from build123d import *

# Parameters (mm, degrees)
SKETCH_1_W      = 289
SKETCH_1_H      = 22.5
EXTRUDE_1_DEPTH = 21
FILLET_1_R      = 9


with BuildPart() as part:
    # 草图1 → 凸台-拉伸1 (new body)
    with BuildSketch(Plane.XY):
        Rectangle(SKETCH_1_W, SKETCH_1_H)
    extrude(amount=EXTRUDE_1_DEPTH)

    # 圆角1
    fillet_1_edges = [part.edges().sort_by_distance(p)[0] for p in [
        (0, 11.25, 0),
    ]]
    fillet(fillet_1_edges, radius=FILLET_1_R)


solid = part.part
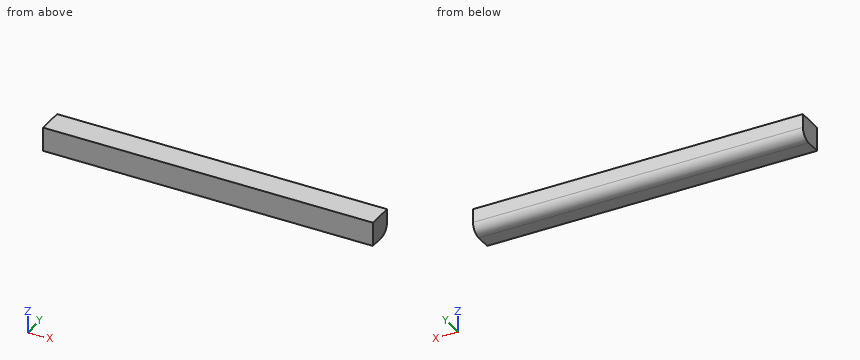
Could you check a few things on this model? Use its own coordinates, in mm. Round coordinates to 2 decimals unless told otherwise and drop trailing zeros. Order: outer loops, then holes, each group sorted by start corner. A loop starts at its lowest first (then second) coordinate and runs counter-clockwise, first axis right, second up. Notation, with made-up numbers: M 17,-32.5 L 59,-32.5 A13 ccw 59,-17.5 Z; hole C 56,-31.75 d10. An arc over 180 degrees is marked long. One line per item, written item: value.
(1) I'm going to push flat-ended pins straight in: P1, Ø4, axis at x = 38.5, z = 4, coming from the +Y side; P2, Ø10, axis at x = -87.5, y = 7, coming from the -Z side. Where does each tip first touch, or does it pass through?
Ans:
P1: stops at y = 10.74
P2: stops at z = 0
(2) Imagine slicing it at B-B (y = 8.75). Write out the boundary of the cut face in (x, z), and give its area (3 significant figures).
Ans:
outline: M -144.5,2.78 L 144.5,2.78 L 144.5,21 L -144.5,21 Z
area: 5,270 mm^2
(3) I need wall thicknesses on line 1 along Z through (x, y) = (-58, 3); line 2 along Z through (x, y) = (-33, 3.25); line 3 along Y through (x, z) = (40.5, 6.25). Which ranges of each line are inside material? Lowest first, please. Write a range as from..to.
Ans:
line 1: z = 0.03..21
line 2: z = 0.06..21
line 3: y = -11.25..10.82
(4) Imagine slicing it at C-C (z = 3). Write out the boundary of the cut face in (x, y).
Ans:
outline: M -144.5,-11.25 L 144.5,-11.25 L 144.5,8.96 L -144.5,8.96 Z
(5) Imagine slicing it at A-A (x = -57.5). Write out the boundary of the cut face in (y, z).
Ans:
outline: M -11.25,0 L 2.25,0 A9 ccw 11.25,9 L 11.25,21 L -11.25,21 Z
